Geometry: final body of the model. Coordinates: model frame, mm. Face numbers are marked on the shaded views. A direction names the side the tool comes from. Round coordinates to 2 decimals unless told otherwise and drop trailing zeros. Order: outer loops, then holes, each group sorted by start corner. A loop starts at its lowest first (then second) coordinate and runs counter-clockwise, first axis right, second up. Notation, with made-up numbers: M 44.25,65.25 L 66.25,65.25 A29 cw 66.25,86.25 Z; hole C 83.25,44 d7. An arc over 180 degrees is marked long. Put each result on its own line as item: value. Start each with the question number.
1) Section B-B, the plane z = 0. Return loops of the section in (x, y), then the cut area to 3 significant figures.
2) Access query for the marked faces 5, 6 and 7. Directions: +Z, -Z, +X, -X, +Y, -Y. A direction counts if a zero-diameter tool reaches every point of the face in a straight line with its end or side. Return the directions, or none.
3) Section A-A, the plane x = 0. Return loops of the section in (y, z).
4) Section D-D, the plane z = -14.5. Return loops of the section in (x, y), then the cut area to 3 significant figures.
5) Draft query along Z for the marked faces 1, 2, 3 and 4. Return one class per face: pulls with the +Z half, pulls with the -Z half, needs draft (parallel to the pull), parting line crosses it, or undercut.
6) Material intervals for probe 1 along Z at (x, y) = (-18.5, 12.75); probe 2 along Z at (x, y) = (0.5, 14.5); probe 3 along X at (y, z) = (13.5, 14), sorted ascending. Write a range as [from, to].
7) Section C-C, the plane y = 5.5. Return loops of the section in (x, z), then the cut area to 3 significant figures.
8) First-contact query: P1, Ø1.5, axis at x = 10.5, y = 6.5, coming from the -Z side; P2, Ø7, axis at x = -14.85, z = -14.85, coming from the -Y side; P3, Ø5, axis at x = -8, z = -2.5, coming from the +Y side; P4, Ø13, axis at x = -14.85, z = 14.85, coming from the -Y side. Flat tips, straight axial feed; report the tip coordinate or a pass-through.
from build123d import *

# Parameters (mm, degrees)
SKETCH1_R                                           = 17
SKETCH1_R_2                                         = 5
BOSS_EXTRUDE1_DEPTH                                 = 8
SKETCH2_W                                           = 42
SKETCH2_H                                           = 42
SKETCH2_R                                           = 5
BOSS_EXTRUDE2_DEPTH                                 = 7
FILLET1_R                                           = 7
CBORE_FOR_M4_HEX_SOCKET_HEAD_CAP_SCREW1_D           = 4.5
CBORE_FOR_M4_HEX_SOCKET_HEAD_CAP_SCREW1_CBORE_D     = 8
CBORE_FOR_M4_HEX_SOCKET_HEAD_CAP_SCREW1_CBORE_DEPTH = 4.4
SKETCH5_R                                           = 13
CUT_EXTRUDE1_DEPTH                                  = 3.5
CUT_EXTRUDE2_START                                  = -3.5
SKETCH6_R                                           = 13
CUT_EXTRUDE2_DEPTH                                  = 3.5


with BuildPart() as part:
    # Sketch1 → Boss-Extrude1 (new body)
    with BuildSketch(Plane(origin=(0, 0, 0), x_dir=(1, 0, 0), z_dir=(0, 1, 0))):
        with Locations(Location((0, 0, 0), (0, 0, 270))):
            Circle(SKETCH1_R)
        with Locations(Location((0, 0, 0), (0, 0, 270))):
            Circle(SKETCH1_R_2, mode=Mode.SUBTRACT)
    extrude(amount=BOSS_EXTRUDE1_DEPTH)

    # Sketch2 → Boss-Extrude2 (add)
    with BuildSketch(Plane(origin=(0, 8, 0), x_dir=(1, 0, 0), z_dir=(0, 1, 0))):
        Rectangle(SKETCH2_W, SKETCH2_H)
        with Locations(Location((0, 0, 0), (0, 0, 270))):
            Circle(SKETCH2_R, mode=Mode.SUBTRACT)
    extrude(amount=BOSS_EXTRUDE2_DEPTH)

    # Fillet1
    fillet1_edges = [part.edges().sort_by_distance(p)[0] for p in [
        (-21, 11.5, -21),
        (-21, 11.5, 21),
        (21, 11.5, 21),
        (21, 11.5, -21),
    ]]
    fillet(fillet1_edges, radius=FILLET1_R)

    # CBORE for M4 Hex Socket Head Cap Screw1 (through all)
    with Locations(Plane(origin=(-14.849242405, 15, -14.849242405), x_dir=(0, 0, 1), z_dir=(0, 1, 0))):
        with Locations((0, 0), (0, 29.69848481), (29.69848481, 29.69848481), (29.69848481, 0)):
            CounterBoreHole(CBORE_FOR_M4_HEX_SOCKET_HEAD_CAP_SCREW1_D / 2, CBORE_FOR_M4_HEX_SOCKET_HEAD_CAP_SCREW1_CBORE_D / 2, CBORE_FOR_M4_HEX_SOCKET_HEAD_CAP_SCREW1_CBORE_DEPTH)

    # Sketch5 → Cut-Extrude1 (cut)
    with BuildSketch(Plane.XZ):
        with Locations(Location((0, 0, 0), (0, 0, 270))):
            Circle(SKETCH5_R)
    extrude(amount=-CUT_EXTRUDE1_DEPTH, mode=Mode.SUBTRACT)

    # Sketch6 → Cut-Extrude2 (cut)
    with BuildSketch(Plane(origin=(0, 15, 0), x_dir=(1, 0, 0), z_dir=(0, 1, 0)).offset(CUT_EXTRUDE2_START)):
        with Locations(Location((0, 0, 0), (0, 0, 90))):
            Circle(SKETCH6_R)
    extrude(amount=CUT_EXTRUDE2_DEPTH, mode=Mode.SUBTRACT)


solid = part.part
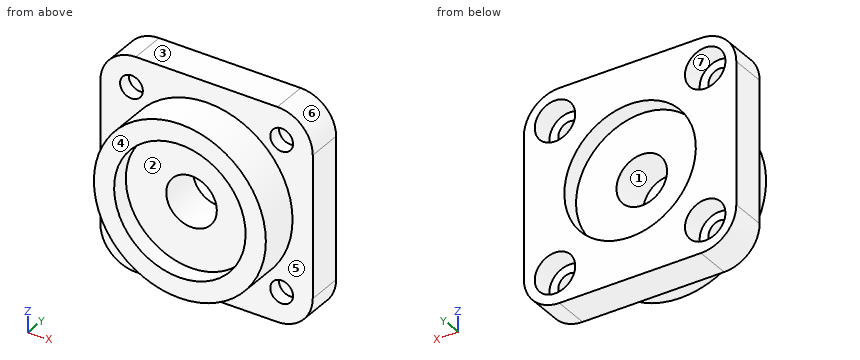
Result sheet:
1. outline: M -21,8 L -17,8 L -17,0 L -13,0 L -13,3.5 L -5,3.5 L -5,11.5 L -13,11.5 L -13,15 L -21,15 Z; M 5,3.5 L 13,3.5 L 13,0 L 17,0 L 17,8 L 21,8 L 21,15 L 13,15 L 13,11.5 L 5,11.5 Z
1. area: 304 mm2
2. face 5: -Y
2. face 6: +Z, +X, +Y, -Y
2. face 7: +Y
3. outline: M 0,-17 L 8,-17 L 8,-21 L 15,-21 L 15,-13 L 11.5,-13 L 11.5,-5 L 3.5,-5 L 3.5,-13 L 0,-13 Z; M 0,13 L 3.5,13 L 3.5,5 L 11.5,5 L 11.5,13 L 15,13 L 15,21 L 8,21 L 8,17 L 0,17 Z
4. outline: M -20.98,8 L -17.07,8 L -17.07,10.6 L -18.83,10.6 L -18.83,15 L -20.98,15 Z; M -12.63,8 L -8.87,8 L -8.87,0 L 8.87,0 L 8.87,8 L 12.63,8 L 12.63,10.6 L 10.86,10.6 L 10.86,15 L -10.86,15 L -10.86,10.6 L -12.63,10.6 Z; M 17.07,8 L 20.98,8 L 20.98,15 L 18.83,15 L 18.83,10.6 L 17.07,10.6 Z
4. area: 342 mm2
5. face 1: undercut
5. face 2: undercut
5. face 3: pulls with the +Z half
5. face 4: needs draft
6. probe 1: z = [-19.36, -16.48], [-13.21, 13.21], [16.48, 19.36]
6. probe 2: z = [-21, -12.99], [12.99, 21]
6. probe 3: x = [-21, -18.76], [-10.94, 10.94], [18.76, 21]
7. outline: C 0,0 d34; hole C 0,0 d10
7. area: 829 mm2
8. P1: stops at z = -13.93
8. P2: stops at y = 8
8. P3: stops at y = 11.5
8. P4: stops at y = 0
